```python
from build123d import *


# Not quite as in the source:
# - a fillet or chamfer that OpenCascade refuses, or shapes differently, is made with other operations: its cross-section is extruded or revolved along the edge and cut away or added


with BuildPart() as f1:
    # F0 (on Front) → F1 (revolve)
    with BuildSketch(Plane.XZ):
        Polygon((0, 9.95), (0, 0), (13, 0), (13, 3), (10, 3), (10, 6.5), (5.5, 6.5), (5.5, 6.95), (4.05, 6.95), (4.05, 9.95), align=None)
    revolve(axis=Axis((0, 0, 4.975), (0, 0, -1)))

    # F2: chamfer of 0.5 on 5 edges, made by hand

    # F2_s1 → F2_t2 (revolve, cut)
    with BuildSketch(Plane.XZ):
        Polygon((12.5, 0), (13, 0.5), (13, 0), align=None)
    revolve(axis=Axis((0, 0, 0), (0, 0, -1)), mode=Mode.SUBTRACT)

    # F2_s3 → F2_t4 (revolve, cut)
    with BuildSketch(Plane.XZ):
        Polygon((13, 2.5), (12.5, 3), (13, 3), align=None)
    revolve(axis=Axis((0, 0, 3), (0, 0, -1)), mode=Mode.SUBTRACT)

    # F2_s5 → F2_t6 (revolve, cut)
    with BuildSketch(Plane.XZ):
        Polygon((10, 6), (9.5, 6.5), (10, 6.5), align=None)
    revolve(axis=Axis((0, 0, 6.5), (0, 0, -1)), mode=Mode.SUBTRACT)


with BuildPart() as f2_tool8:
    # F2_s9 → F2_t10 (revolve)
    with BuildSketch(Plane.XZ):
        Polygon((5.5, 6.45), (5, 6.95), (5.5, 6.95), align=None)
    revolve(axis=Axis((0, 0, 6.95), (0, 0, -1)))

    split(bisect_by=Plane.XY.offset(6.5), keep=Keep.TOP)


with BuildPart() as f1_1:
    add(f1.part)

    # F2_t7: cut F2_tool8
    add(f2_tool8.part, mode=Mode.SUBTRACT)

    # F2_s12 → F2_t13 (revolve, cut)
    with BuildSketch(Plane.XZ):
        Polygon((4.05, 9.45), (3.55, 9.95), (4.05, 9.95), align=None)
    revolve(axis=Axis((0, 0, 9.95), (0, 0, -1)), mode=Mode.SUBTRACT)


solid = f1_1.part
```
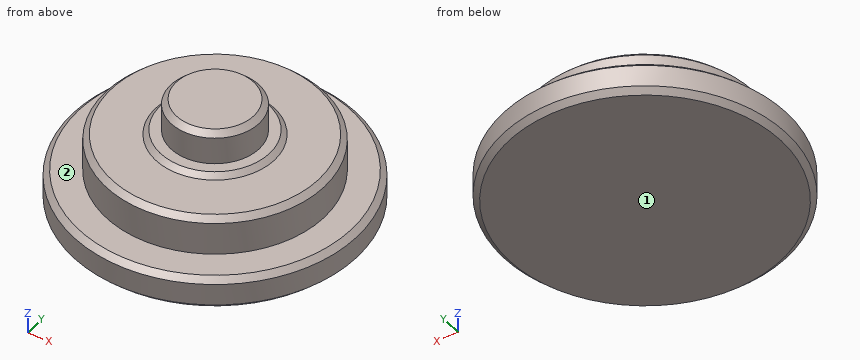
Here's how the part is built. I have some questions about the finished solid (model axes, mm). Face numbers are marked on the shaded views. A direction names the side the tool comes from. Give positions to 0.01 mm unless a question says otherwise; leave off trailing zeros. Loops run counter-clockwise (first coordinate to the right, second up) from the corner with the lowest first, then second, coordinate; pieces in that order, holes last. Notation, with made-up numbers: M 62,33 L 85,33 A28 cw 85,61 Z; hole C 75,-14.5 d4. An arc over 180 degrees is marked long. Use one line per item in the form item = value. Start each with the question number.
Q1. Will these pins go through, and if not, where does the flat tip stop? pin 1 Ø5 at (x, z) = (8.5, 3.5) entering from +Y; pin 2 Ø5 at (x, z) = (9.5, 2) entering from +Y; pin 3 Ø1.5 at (x, y) = (6, 2.5) entering from +Z.
Q2. Which directions (+Z, -Z, +X, -X, +Y, -Y) give clear straight access to the entire face, cutting with the end or side of a thin tool? Please do the marked faces 1 and 2.
Q3. If we section it at C-C (z = 4.75): Write out the boundary of the cut face in (x, y), then the cut area to 3 significant figures.
Q4. I need wall thicknesses on line 1 along Z through (x, y) = (-3.5, -6.5); line 2 along Z through (x, y) = (-11, 1); line 3 along Y through (x, z) = (7.75, 3.75). Which ranges of each line are inside material? Lowest first, please.
Q5. If we section it at D-D (z = 7.5): Write out the boundary of the cut face in (x, y).
Q6. If we section it at A-A (y = 0): Write out the boundary of the cut face in (x, z), then the cut area to 3 significant figures.
Taken from the geometry:
q1.pin_1 = 11.42
q1.pin_2 = 10.95
q1.pin_3 = 6.5
q2.face_1 = -Z, +X, -X, +Y, -Y
q2.face_2 = +Z
q3.outline = C 0,0 d20
q3.area = 314 mm^2
q4.line_1 = 0 to 6.5
q4.line_2 = 0 to 3
q4.line_3 = -6.32 to 6.32
q5.outline = C 0,0 d8.1
q6.outline = M -13,0.5 L -12.5,0 L 12.5,0 L 13,0.5 L 13,2.5 L 12.5,3 L 10,3 L 10,6 L 9.5,6.5 L 5.45,6.5 L 5,6.95 L 4.05,6.95 L 4.05,9.45 L 3.55,9.95 L -3.55,9.95 L -4.05,9.45 L -4.05,6.95 L -5,6.95 L -5.45,6.5 L -9.5,6.5 L -10,6 L -10,3 L -12.5,3 L -13,2.5 Z
q6.area = 176 mm^2
